```python
from build123d import *

# Parameters (mm, degrees)
F0_W     = 130
F0_H     = 120
F1_DEPTH = 34
F2_ANGLE = 30
F3_W     = 98
F3_H     = 78
F4_DEPTH = 25
F6_DEPTH = 16
F7_R     = 0.95
F8_DEPTH = 8


with BuildPart() as f1:
    # F0 (on Top) → F1 (new body)
    with BuildSketch(Plane.XY):
        Rectangle(F0_W, F0_H)
    extrude(amount=F1_DEPTH)

    # F0 (on Top) → F2 (revolve)
    with BuildSketch(Plane.XY):
        Rectangle(F0_W, F0_H)
    revolve(axis=Axis((0, -60, 0), (-1, 0, 0)), revolution_arc=F2_ANGLE)

    # F3 (on face) → F4 (cut)
    with BuildSketch(Plane(origin=(0, -15, -25.9807621135), x_dir=(1, 0, 0), z_dir=(0, -0.5, -0.8660254038))):
        with Locations((0, -8.0384757729)):
            Rectangle(F3_W, F3_H)
    extrude(amount=-F4_DEPTH, mode=Mode.SUBTRACT)

    # F5 (on face) → F6 (cut)
    with BuildSketch(Plane(origin=(-65, 0, 0), x_dir=(0, -1, 0), z_dir=(-1, 0, 0))):
        Polygon((10.832704407, -16.8397459622), (36.8134665205, -1.8397459622), (29.3134665205, 11.1506350946), (3.332704407, -3.8493649054), align=None)
    extrude(amount=-F6_DEPTH, mode=Mode.SUBTRACT)

    # F7 (on face) → F8 (cut)
    with BuildSketch(Plane(origin=(0, -15, -25.9807621135), x_dir=(1, 0, 0), z_dir=(0, -0.5, -0.8660254038))):
        with Locations((57, 41.4615242271)):
            Circle(F7_R)
        with Locations((-57, 41.4615242271)):
            Circle(F7_R)
        with Locations((-57, -57.5384757729)):
            Circle(F7_R)
        with Locations((57, -57.5384757729)):
            Circle(F7_R)
    extrude(amount=-F8_DEPTH, mode=Mode.SUBTRACT)


solid = f1.part
```
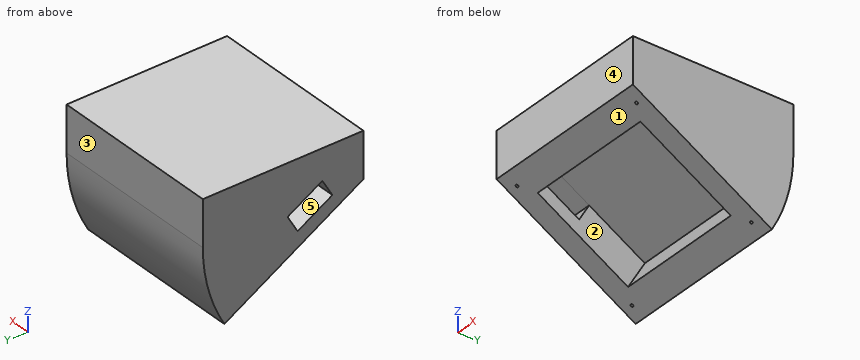
Verification items for the finished model (mm, model axes). Face numbers are marked on the shaded views. A direction names the side the tool comes from. Round coordinates to 2 decimals unless told otherwise and drop trailing zeros. Write each loop counter-clockwise with the first axis right and the second up, starting at its lowest first coordinate (ties: lowest second). Pieces come first, ordered by that corner, then holes.
1. Section check D-D on z = 9. Enter the section's corners in (x, y), plus the area to 3 significant figures.
2. Section check A-A on z = -13.5. Enter the section's corners in (x, y).
3. Section check C-C on y = -13.5. Enter the section's corners in (x, z), plus the area to 3 significant figures.
4. Draft check along Z on the marked faces 1, 2 and 3. Enter one of: +Z half, -Z half, draft (parallel to the pull), parting line (faces both ways), or undercut.
5. Scan lines: L1, parallel to X at y = -36, z = -9; L2, parallel to Y at x = -38, z = 7; L3, parallel to Z at x = -17, y = 31. Record each from-to range of solid material in increasing order.
6. Section check B-B on x = 27.5. Enter the section's corners in (y, z), plus the area to 3 significant figures.
7. Gauge pin test, flat ends, axial feed: P1, Ø12, axis at x = -9, z = -9, coming from the -Y side; P2, Ø1, axis at x = -38, y = -1, coming from the -Z side; P3, Ø1, axis at x = -12, y = 35, coming from the -Z side; P4, Ø5, axis at y = -31.5, z = -18, coming from the -X side. Record the tip position at first contact, or that the pin passes through.
8. Access from +Z, -Z, +X, -X, +Y, -Y to the whole of each face (thin tool, end or side, straight path). Record for the marked faces 4 and 5.
Answer:
1. outline: (-65, -60) - (65, -60) - (65, 60) - (-65, 60) - (-65, -25.59) - (49, -25.59) - (49, -30.56) - (-65, -30.56) - close
1. area: 15,000 mm2
2. outline: (-65, -36.62) - (-49, -36.62) - (-49, -16.62) - (-65, -16.62) - close; (-65, -8.9) - (-49, -8.9) - (-49, 13.38) - (49, 13.38) - (49, -36.62) - (65, -36.62) - (65, 59.24) - (-65, 59.24) - close
3. outline: (-65, -26.85) - (-49, -26.85) - (-49, -15.3) - (-65, -15.3) - close; (-65, 2.02) - (49, 2.02) - (49, -26.85) - (65, -26.85) - (65, 34) - (-65, 34) - close
3. area: 4,800 mm2
4. face 1: -Z half
4. face 2: undercut
4. face 3: draft
5. L1: x = -65 to -49, 49 to 65
5. L2: y = -60 to -31.71, -22.12 to 60
5. L3: z = -52.54 to -40.38, -23.67 to 34
6. outline: (-60, 0) - (-41.81, -10.5) - (-29.31, 11.15) - (38.24, -27.85) - (25.74, -49.5) - (43.92, -60) arc R120 ccw to (60, 0) - (60, 34) - (-60, 34) - close
6. area: 5,900 mm2
7. P1: stops at y = -54.8
7. P2: stops at z = -5.48
7. P3: stops at z = -55.14
7. P4: stops at x = -65
8. face 4: +Z, -Z, +X, -X, -Y
8. face 5: -X
